from build123d import *

# Parameters (mm, degrees)
SKETCH2_R           = 2
BOSS_EXTRUDE1_DEPTH = 7.5
CIRPATTERN1_COUNT   = 8
SKETCH3_R           = 1.8
SKETCH3_R_2         = 1.5
BOSS_EXTRUDE2_DEPTH = 0.005


with BuildPart() as part:
    # Sketch1 → Revolve1 (revolve)
    with BuildSketch(Plane.XY):
        with BuildLine():
            Line((0, 0), (0, 62))
            Line((0, 62), (13.5, 62))
            ThreePointArc((13.5, 62), (14.207106781, 61.707106781), (14.5, 61))
            Line((14.5, 61), (14.5, 55.005))
            Line((14.5, 55.005), (11, 55.005))
            Line((11, 55.005), (11, 54.995))
            Line((11, 54.995), (14.5, 54.995))
            Line((14.5, 54.995), (14.5, 49))
            Line((14.5, 49), (11, 49))
            Line((11, 49), (11, 47))
            Line((11, 47), (14.5, 47))
            Line((14.5, 47), (14.5, 44.5))
            Line((14.5, 44.5), (12.5, 44.5))
            Line((12.5, 44.5), (12.5, 37))
            Line((12.5, 37), (11, 37))
            Line((11, 37), (11, 0))
            Line((11, 0), (0, 0))
        make_face()
    revolve(axis=Axis((0, 0, 0), (0, -1, 0)))

    # Sketch2 → Boss-Extrude1 (add)
    with BuildSketch(Plane.XZ.offset(-44.5)):
        with Locations((0, 12.5)):
            Circle(SKETCH2_R)
    boss_extrude1 = extrude(amount=BOSS_EXTRUDE1_DEPTH)

    # CirPattern1: Boss-Extrude1 ×8 about axis
    cirpattern1_axis = Axis((0, 0, 0), (0, 1, 0))
    for i in range(1, CIRPATTERN1_COUNT):
        add(boss_extrude1.rotate(cirpattern1_axis, i * 360 / CIRPATTERN1_COUNT))

    # Sketch3 → Boss-Extrude2 (add)
    with BuildSketch(Plane(origin=(0, 62, 0), x_dir=(1, 0, 0), z_dir=(0, 1, 0))):
        Circle(SKETCH3_R)
        Circle(SKETCH3_R_2, mode=Mode.SUBTRACT)
        with BuildLine():
            Line((-4.330127019, -2.5), (-4.58993464, -2.65))
            ThreePointArc((-4.58993464, -2.65), (-5.3, 0), (-4.58993464, 2.65))
            Line((-4.58993464, 2.65), (-4.330127019, 2.5))
            ThreePointArc((-4.330127019, 2.5), (-5, 0), (-4.330127019, -2.5))
        make_face()
        with BuildLine():
            Line((-3.031088913, -1.75), (-3.290896534, -1.9))
            ThreePointArc((-3.290896534, -1.9), (-3.8, 0), (-3.290896534, 1.9))
            Line((-3.290896534, 1.9), (-3.031088913, 1.75))
            ThreePointArc((-3.031088913, 1.75), (-3.5, 0), (-3.031088913, -1.75))
        make_face()
        with BuildLine():
            Line((-5.629165125, -3.25), (-5.888972746, -3.4))
            ThreePointArc((-5.888972746, -3.4), (-6.8, 0), (-5.888972746, 3.4))
            Line((-5.888972746, 3.4), (-5.629165125, 3.25))
            ThreePointArc((-5.629165125, 3.25), (-6.5, 0), (-5.629165125, -3.25))
        make_face()
        with BuildLine():
            Line((-6.92820323, -4), (-7.188010851, -4.15))
            ThreePointArc((-7.188010851, -4.15), (-8.3, 0), (-7.188010851, 4.15))
            Line((-7.188010851, 4.15), (-6.92820323, 4))
            ThreePointArc((-6.92820323, 4), (-8, 0), (-6.92820323, -4))
        make_face()
        with BuildLine():
            Line((6.92820323, 4), (7.188010851, 4.15))
            ThreePointArc((7.188010851, 4.15), (8.3, 0), (7.188010851, -4.15))
            Line((7.188010851, -4.15), (6.92820323, -4))
            ThreePointArc((6.92820323, -4), (8, 0), (6.92820323, 4))
        make_face()
        with BuildLine():
            Line((5.629165125, 3.25), (5.888972746, 3.4))
            ThreePointArc((5.888972746, 3.4), (6.8, 0), (5.888972746, -3.4))
            Line((5.888972746, -3.4), (5.629165125, -3.25))
            ThreePointArc((5.629165125, -3.25), (6.5, 0), (5.629165125, 3.25))
        make_face()
        with BuildLine():
            Line((4.330127019, 2.5), (4.58993464, 2.65))
            ThreePointArc((4.58993464, 2.65), (5.3, 0), (4.58993464, -2.65))
            Line((4.58993464, -2.65), (4.330127019, -2.5))
            ThreePointArc((4.330127019, -2.5), (5, 0), (4.330127019, 2.5))
        make_face()
        with BuildLine():
            Line((3.031088913, 1.75), (3.290896534, 1.9))
            ThreePointArc((3.290896534, 1.9), (3.8, 0), (3.290896534, -1.9))
            Line((3.290896534, -1.9), (3.031088913, -1.75))
            ThreePointArc((3.031088913, -1.75), (3.5, 0), (3.031088913, 1.75))
        make_face()
    extrude(amount=BOSS_EXTRUDE2_DEPTH)


solid = part.part
CAD build for the part. Positions are in the model's coordinates, mm. A direction names the side the tool comes from. Give positions to 0.01 mm unless a question says otherwise; leave off trailing zeros. Loops run counter-clockwise (first coordinate to the right, second up) from the corner with the lowest first, then second, coordinate; pieces in that order, holes last. Notation, with made-up numbers: M 53.5,49.25 L 105.5,49.25 A25 ccw 105.5,68.25 Z; hole C 13,9.5 d1. An arc over 180 degrees is marked long. Answer in a Markdown table with one row per item. Add a question column.
Item 1: Probe probe 1 along Y at (x, z) = (2.75, -2.75); probe 2 along Z at (x, y) = (10, 36.5); probe 3 along Z at (x, y) = (-0.5, 46). List the from-to ranges inside material, lowest first.
Item 2: Band-saw the part on A-A on y = 34. Give the cut face in (x, z).
Item 3: Drop flat-ended pins along their axis: P1, Ø6, axis at y = 34.5, z = 8.5, coming from the -X side; P2, Ø2, axis at x = 0, y = 11.5, coming from the +Z side; P3, Ø8, axis at x = 2, y = 39.5, coming from the +Z side; P4, Ø1.3, axis at x = -6, z = 13, coming from the -Y side. Give the stop position or say it passes through.
Item 4: Band-saw the part on B-B on y = 53. Give the cut face in (x, z), then the cut area to 3 significant figures.
Item 5: Tool access for faces 1 (the face through (4.746, 40.698, -11.564)), 2 (the face through (-10.285, 40.802, -10.22)), 3 (the face through (0, 0, 0)): list every direction of +Z, -Z, +X, -X, +Y, -Y with a clear straight run to the whole face (end or side of a thin tool).
Item 6: Mould opens along Z. For faces 4 (the face through (6.691, 57.961, -12.864)), 5 (the face through (-11.533, 40.698, 4.821)), 6 (the face through (5, 44.5, -12)) say: +Z half, -Z half, draft (parallel to the pull), parting line (faces both ways), or undercut.
Reply:
| question | item | result |
|---|---|---|
| 1 | probe 1 | y = 0 to 62 |
| 1 | probe 2 | z = -4.58 to 4.58 |
| 1 | probe 3 | z = -14.49 to 14.49 |
| 2 | outline | C 0,0 d22 |
| 3 | P1 | stops at x = -10.84 |
| 3 | P2 | stops at z = 11 |
| 3 | P3 | stops at z = 14.5 |
| 3 | P4 | stops at y = 44.5 |
| 4 | outline | C 0,0 d29 |
| 4 | area | 661 mm^2 |
| 5 | face 1 | -Z, -Y |
| 5 | face 2 | -Y |
| 5 | face 3 | +Z, -Z, +X, -X, -Y |
| 6 | face 4 | parting line |
| 6 | face 5 | undercut |
| 6 | face 6 | draft |
